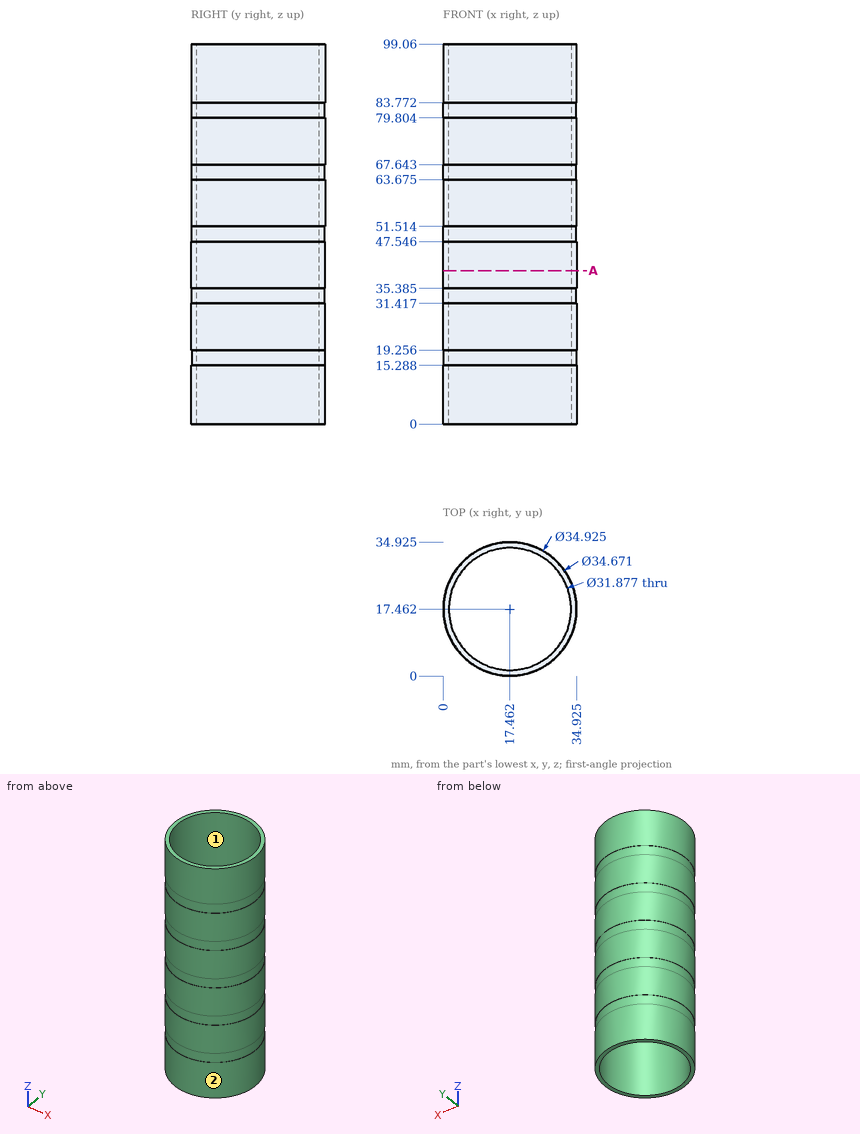
Can you work these out from the drawing? Everything is in mm from the part's minimum corner. Coordinates: 2 decimals unless noted, no trailing zeros. Loops run counter-clockwise (first coordinate to the right, second up) from the corner with the lowest first, then second, coordinate; pieces in that order, holes last.
1) I need wall thicknesses on probe 1 along Y at (x, z) = (17, 13.5) (1 decimal); probe 2 along X at (y, z) = (12.5, 64) (1 decimal); probe 3 along Y at (x, z) = (16, 67). Which ranges of each line are inside material? Lowest first, please.
2) Thinking about a two-plate mould opening in X: for the marked faces 1 and 2, which applies, pulls with the +X half, pulls with the -X half, needs draft (parallel to the pull), parting line crosses it, or undercut?
3) Imagine slicing it at A-A on z = 40. List the corners of the cut face in (x, y) for me (1 decimal), plus the area to 3 significant figures.
4) For pin 1 (1.5 mm diameter, centred on y = 24, z = 47, fed in from -X); pin 2 (17.5 mm diameter, centred on x = 23.5, y = 9, fed in from +Z); pin 3 (6 mm diameter, centred on y = 6.5, z = 29, fed in from -X); pin 4 (1 mm diameter, centred on x = 23.5, z = 85, fed in from +Y), each with a flat end and sliding along its axis, tell me the tip position at first contact or that it passes through.
Completed:
1. probe 1: y = 0 to 1.5, 33.4 to 34.9
1. probe 2: x = 0.9 to 2.3, 32.6 to 34.1
1. probe 3: y = 0.19 to 1.59, 33.33 to 34.74
2. face 1: undercut
2. face 2: parting line crosses it
3. outline: circle Ø34.9 at (17.5, 17.5); hole circle Ø31.9 at (17.5, 17.5)
3. area: 160 mm2
4. pin 1: stops at x = 0.99
4. pin 2: stops at z = 99.06
4. pin 3: stops at x = 1.92
4. pin 4: stops at y = 34.02
